Source: CAD feature listing. Evaluate the final solid. Frame: model axes, mm. A direction names the side the tool comes from. Give positions to 0.01 mm unless a question says otherwise; leave off trailing zeros. Loops run counter-clockwise (first coordinate to the right, second up) from the corner with the lowest first, then second, coordinate; pieces in that order, holes last. Notation, with made-up numbers: M 54.5,-3 L 85.5,-3 A29 ccw 85.5,36 Z; hole C 10.5,-5 d5. An arc over 180 degrees is marked long. Write item = value, one per line.
from build123d import *

# Parameters (mm, degrees)
PAD_DEPTH             = 5
SKETCH001_W           = 23
SKETCH001_H           = 12
POCKET_DEPTH          = 5
POLARPATTERN_COUNT    = 2
POLARPATTERN001_COUNT = 6


with BuildPart() as part:
    # Sketch → Pad (new body)
    with BuildSketch(Plane.XY):
        Polygon((-25, -43.30127), (25, -43.30127), (50, 0), (25, 43.30127), (-25, 43.30127), (-50, 0), align=None)
    extrude(amount=PAD_DEPTH)

    # Sketch001 (on Face8 of Pad) → Pocket (cut)
    with BuildSketch(Plane.XY.offset(5)):
        with Locations((0, 32.30127)):
            Rectangle(SKETCH001_W, SKETCH001_H)
    pocket = extrude(amount=-POCKET_DEPTH, mode=Mode.SUBTRACT)

    # PolarPattern: Pocket ×2 about axis
    polarpattern_axis = Axis((0, 0, 5), (0, 0, 1))
    for i in range(1, POLARPATTERN_COUNT):
        add(pocket.rotate(polarpattern_axis, i * 360 / POLARPATTERN_COUNT), mode=Mode.SUBTRACT)

    # PolarPattern001: Pocket ×6 about axis
    polarpattern001_axis = Axis((0, 0, 0), (0, 0, 1))
    for i in range(1, POLARPATTERN001_COUNT):
        add(pocket.rotate(polarpattern001_axis, i * 360 / POLARPATTERN001_COUNT), mode=Mode.SUBTRACT)


solid = part.part
1. Reachability of faces 1 (the flat face through (-22.151, 26.068, 2.535)), 2 (the flat face through (-1, 1, 0)) from +Z, -Z, +X, -X, +Y, -Y: full face, straight path, thin tool, end or side. Return the list, or none.
Derived:
face_1 = +Z, -Z
face_2 = -Z, +X, -X, +Y, -Y
2. Cut plane D-D, the plane y = 34.5. Return the cut outline in (x, z).
Derived:
outline = M -30.08,0 L -11.5,0 L -11.5,5 L -30.08,5 Z; M 11.5,0 L 30.08,0 L 30.08,5 L 11.5,5 Z
3. Cut plane A-A, the plane x = -3. Return the cut outline in (y, z).
Derived:
outline = M -43.3,0 L -38.3,0 L -38.3,5 L -43.3,5 Z; M -26.3,0 L 26.3,0 L 26.3,5 L -26.3,5 Z; M 38.3,0 L 43.3,0 L 43.3,5 L 38.3,5 Z
4. Cut plane B-B, the plane y = 6. Return the cut outline in (x, z), then the cut area to 3 significant figures.
Derived:
outline = M -46.54,0 L -33.39,0 L -33.39,5 L -46.54,5 Z; M -26.91,0 L 26.91,0 L 26.91,5 L -26.91,5 Z; M 33.39,0 L 46.54,0 L 46.54,5 L 33.39,5 Z
area = 400 mm²
5. Material intervals for probe 1 along Y at (x, z) = (2, 0.6); probe 2 along X at (y, z) = (5, 3.85); probe 3 along Y at (x, z) = (30.5, 2.45) (3 decimals), sorted ascending. Write a range as from..to.
Derived:
probe_1 = -43.3..-38.3, -26.3..26.3, 38.3..43.3
probe_2 = -47.11..-31.66, -27.48..27.48, 31.66..47.11
probe_3 = -33.775..-23.775, -4.33..4.33, 23.775..33.775
6. First-contact query: pin 1 Ø2.5 at (y, z) = (32.5, 3.5) entering from +X; pin 2 Ø2.5 at (y, z) = (35, 2.5) entering from -X; pin 3 Ø1.5 at (y, z) = (-31, 2.5) entering from -X. Flat tips, straight axial feed; report the tip coordinate or a pass-through.
Derived:
pin_1 = 31.96
pin_2 = -30.51
pin_3 = -32.54
7. Pull-direction query (X, two-part tool) for faces 3 (the flat face through (-33.09, -19.29, 2.54)), 4 (the flat face through (0, 26.301, 3)), 5 (the flat face through (37.3, -22, 2.5)), 6 (the flat face through (-1, 1, 5)); classes: +X half, -X half, draft (parallel to the pull), parting line (faces both ways), or undercut.
Derived:
face_3 = undercut
face_4 = undercut
face_5 = +X half
face_6 = draft
8. Cut plane C-C, the plane z = 2. Count the separate pieces of the cut face and the enclosed holes in it, then the cut area to 3 significant figures.
Derived:
separate_pieces = 1
enclosed_holes = 6
area = 4,840 mm²
